```python
from build123d import *

# Parameters (mm, degrees)
SKETCH1_W             = 25.4
SKETCH1_H             = 25.4
BOSS_EXTRUDE1_DEPTH   = 6.35
F_8_32_TAPPED_HOLE5_D = 3.4544
F_6_32_TAPPED_HOLE1_D = 2.7051


with BuildPart() as part:
    # Sketch1 → Boss-Extrude1 (new body)
    with BuildSketch(Plane(origin=(0, 0, 0), x_dir=(0, 0, -1), z_dir=(1, 0, 0))):
        with Locations((12.7, -12.7)):
            Rectangle(SKETCH1_W, SKETCH1_H)
    extrude(amount=BOSS_EXTRUDE1_DEPTH)

    # #8-32 Tapped Hole5 (through all)
    with Locations(Plane.ZY):
        with Locations((-20.32, -20.32), (-20.32, -5.08), (-5.08, -5.08), (-5.08, -20.32)):
            Hole(F_8_32_TAPPED_HOLE5_D / 2)

    # #6-32 Tapped Hole1 (through all)
    with Locations(Plane.ZY):
        with Locations((-12.7, -12.7)):
            Hole(F_6_32_TAPPED_HOLE1_D / 2)


solid = part.part
```
Geometry check sheet. Reference: the model listing, model coordinates, mm. Round coordinates to 2 decimals unless told otherwise and drop trailing zeros. Loops run counter-clockwise (first coordinate to the right, second up) from the corner with the lowest first, then second, coordinate; pieces in that order, holes last. Notation, with made-up numbers: (-19, -7.75) - (9, -7.75) arc R11 cw to (9, 10.25) - close; hole circle Ø5 at (55, -39.75). An arc over 180 degrees is marked (long way). Write item = value, one per line. Start each with the question number.
1. Mould release check, pull along Z, two halves, no side actions. Record for faces 1 (the face through (3, -13, 0)), 2 (the face through (6.35, -13, -15)), 3 (the face through (3.219, -5.004, -18.594)), 4 (the face through (3, -13, -25.4)): released by +Z, released by -Z, zero draft, split by the parting line, or undercut.
2. Thickness scan on line 1 (Y direction, x = 5, z = -5.08); line 2 (Y direction, x = 3.25, z = -12.7); line 3 (Z direction, x = 5.75, y = -19.75). Record the ranges inside material, lowest first.
3. Section check C-C on z = -5.08. Enter the section's corners in (x, y), then the cut area to 3 significant figures.
4. Section check A-A on y = -12.7. Enter the section's corners in (x, z), then the cut area to 3 significant figures.
5. Section check B-B on x = 5.5. Enter the section's corners in (y, z), then the cut area to 3 significant figures.
6. Section check D-D on y = -6. Enter the section's corners in (x, z), then the cut area to 3 significant figures.
Working result:
q1.face_1 = released by +Z
q1.face_2 = zero draft
q1.face_3 = undercut
q1.face_4 = released by -Z
q2.line_1 = -25.4 to -22.05, -18.59 to -6.81, -3.35 to 0
q2.line_2 = -25.4 to -14.05, -11.35 to 0
q2.line_3 = -25.4 to -21.95, -18.69 to -6.71, -3.45 to 0
q3.outline = (0, -25.4) - (6.35, -25.4) - (6.35, -22.05) - (0, -22.05) - close; (0, -18.59) - (6.35, -18.59) - (6.35, -6.81) - (0, -6.81) - close; (0, -3.35) - (6.35, -3.35) - (6.35, 0) - (0, 0) - close
q3.area = 117 mm^2
q4.outline = (0, -25.4) - (6.35, -25.4) - (6.35, -14.05) - (0, -14.05) - close; (0, -11.35) - (6.35, -11.35) - (6.35, 0) - (0, 0) - close
q4.area = 144 mm^2
q5.outline = (-25.4, -25.4) - (0, -25.4) - (0, 0) - (-25.4, 0) - close; hole circle Ø3.45 at (-20.32, -20.32); hole circle Ø3.45 at (-20.32, -5.08); hole circle Ø2.71 at (-12.7, -12.7); hole circle Ø3.45 at (-5.08, -20.32); hole circle Ø3.45 at (-5.08, -5.08)
q5.area = 602 mm^2
q6.outline = (0, -25.4) - (6.35, -25.4) - (6.35, -21.78) - (0, -21.78) - close; (0, -18.86) - (6.35, -18.86) - (6.35, -6.54) - (0, -6.54) - close; (0, -3.62) - (6.35, -3.62) - (6.35, 0) - (0, 0) - close
q6.area = 124 mm^2
